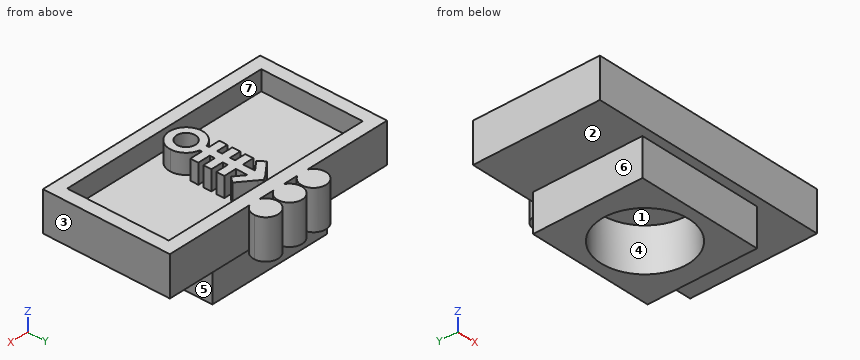
from build123d import *

# Parameters (mm, degrees)
F1_DEPTH = 3.175
F2_W     = 17.018
F2_H     = 8.128
F3_DEPTH = 1.5875
F4_W     = 10.05
F4_H     = 8.76
F5_DEPTH = 3
F6_R     = 3.5
F7_DEPTH = 3.5
F8_R     = 0.75
F8_W     = 0.64
F8_H     = 0.64
F8_W_2   = 1.0036083104
F8_W_3   = 0.8963916896
F8_H_2   = 0.4
F9_DEPTH = 1.5875


with BuildPart() as f1:
    # F0 (on Top) → F1 (new body)
    with BuildSketch(Plane.XY):
        with BuildLine():
            Line((-12.0608898944, 10.16), (-19.05, 10.16))
            Line((-19.05, 10.16), (-19.05, 0))
            Line((-19.05, 0), (0, 0))
            Line((0, 0), (0, 10.16))
            Line((0, 10.16), (-6.9891101056, 10.16))
            ThreePointArc((-6.9891101056, 10.16), (-7.425, 10.06), (-7.8608898944, 10.16))
            Line((-7.8608898944, 10.16), (-9.0891101056, 10.16))
            ThreePointArc((-9.0891101056, 10.16), (-9.525, 10.06), (-9.9608898944, 10.16))
            Line((-9.9608898944, 10.16), (-11.1891101056, 10.16))
            ThreePointArc((-11.1891101056, 10.16), (-11.625, 10.06), (-12.0608898944, 10.16))
        make_face()
        with BuildLine():
            ThreePointArc((-10.625, 11.06), (-12.1560885546, 11.9073163206), (-12.0608898944, 10.16))
            Line((-12.0608898944, 10.16), (-11.1891101056, 10.16))
            ThreePointArc((-11.1891101056, 10.16), (-10.7776836794, 10.5289114454), (-10.625, 11.06))
        make_face()
        with BuildLine():
            Line((-11.1891101056, 10.16), (-12.0608898944, 10.16))
            ThreePointArc((-12.0608898944, 10.16), (-11.625, 10.06), (-11.1891101056, 10.16))
        make_face()
        with BuildLine():
            ThreePointArc((-8.525, 11.06), (-10.0560885546, 11.9073163206), (-9.9608898944, 10.16))
            Line((-9.9608898944, 10.16), (-9.0891101056, 10.16))
            ThreePointArc((-9.0891101056, 10.16), (-8.6776836794, 10.5289114454), (-8.525, 11.06))
        make_face()
        with BuildLine():
            Line((-9.0891101056, 10.16), (-9.9608898944, 10.16))
            ThreePointArc((-9.9608898944, 10.16), (-9.525, 10.06), (-9.0891101056, 10.16))
        make_face()
        with BuildLine():
            ThreePointArc((-7.8608898944, 10.16), (-7.425, 10.06), (-6.9891101056, 10.16))
            Line((-6.9891101056, 10.16), (-7.8608898944, 10.16))
        make_face()
        with BuildLine():
            Line((-7.8608898944, 10.16), (-6.9891101056, 10.16))
            ThreePointArc((-6.9891101056, 10.16), (-6.5776836794, 10.5289114454), (-6.425, 11.06))
            ThreePointArc((-6.425, 11.06), (-7.9560885546, 11.9073163206), (-7.8608898944, 10.16))
        make_face()
    extrude(amount=F1_DEPTH)

    # F2 (on face) → F3 (cut)
    with BuildSketch(Plane.XY.offset(3.175)):
        with Locations((-9.525, 5.08)):
            Rectangle(F2_W, F2_H)
    extrude(amount=-F3_DEPTH, mode=Mode.SUBTRACT)

    # F4 (on face) → F5 (join)
    with BuildSketch(Plane(origin=(0, 0, 0), x_dir=(1, 0, 0), z_dir=(0, 0, -1))):
        with Locations((-9.525, -5.08)):
            Rectangle(F4_W, F4_H)
    extrude(amount=F5_DEPTH)

    # F6 (on face) → F7 (cut)
    with BuildSketch(Plane(origin=(0, 0, -3), x_dir=(1, 0, 0), z_dir=(0, 0, -1))):
        with Locations((-9.525, -5.08)):
            Circle(F6_R)
    extrude(amount=-F7_DEPTH, mode=Mode.SUBTRACT)

    # F8 (on face) → F9 (join, through all)
    with BuildSketch(Plane.XY.offset(1.5875)):
        with BuildLine():
            ThreePointArc((-9.8986083104, 4.0632728435), (-10.3368278084, 1.6873732761), (-8.175, 2.766))
            ThreePointArc((-8.175, 2.766), (-8.4804597229, 3.6212400888), (-9.2586083104, 4.0894558805))
            ThreePointArc((-9.2586083104, 4.0894558805), (-9.5801836824, 4.1148716622), (-9.8986083104, 4.0632728435))
        make_face()
        with Locations((-9.525, 2.766)):
            Circle(F8_R, mode=Mode.SUBTRACT)
        with BuildLine():
            ThreePointArc((-9.8986083104, 4.0632728435), (-9.5801836824, 4.1148716622), (-9.2586083104, 4.0894558805))
            Line((-9.2586083104, 4.0894558805), (-9.2586083104, 4.266))
            Line((-9.2586083104, 4.266), (-9.8986083104, 4.266))
            Line((-9.8986083104, 4.266), (-9.8986083104, 4.0632728435))
        make_face()
        with Locations((-9.5786083104, 4.586)):
            Rectangle(F8_W, F8_H)
        with Locations((-8.7568041552, 4.586)):
            Rectangle(F8_W_2, F8_H)
        with Locations((-10.3468041552, 4.586)):
            Rectangle(F8_W_3, F8_H)
        with Locations((-9.5786083104, 5.106)):
            Rectangle(F8_W, F8_H_2)
        with Locations((-9.5786083104, 5.626)):
            Rectangle(F8_W, F8_H)
        with Locations((-8.7568041552, 5.626)):
            Rectangle(F8_W_2, F8_H)
        with Locations((-10.3468041552, 5.626)):
            Rectangle(F8_W_3, F8_H)
        with Locations((-9.5786083104, 6.146)):
            Rectangle(F8_W, F8_H_2)
        with Locations((-9.5786083104, 6.666)):
            Rectangle(F8_W, F8_H)
        with Locations((-8.7568041552, 6.666)):
            Rectangle(F8_W_2, F8_H)
        with Locations((-10.3468041552, 6.666)):
            Rectangle(F8_W_3, F8_H)
        Polygon((-9.8986083104, 6.986), (-9.2586083104, 6.986), (-9.2586083104, 7.9498032218), (-9.2586083104, 8.763), (-9.8986083104, 8.763), (-9.8986083104, 7.9498032218), align=None)
        Polygon((-9.2586083104, 8.763), (-9.2586083104, 7.9498032218), (-8.4652456, 7.3151130535), (-8.0685642448, 7.8109647475), align=None)
        Polygon((-10.6919710208, 7.3151130535), (-9.8986083104, 7.9498032218), (-9.8986083104, 8.763), (-11.088652376, 7.8109647475), align=None)
        Polygon((-9.8986083104, 8.763), (-9.2586083104, 8.763), (-9.525, 8.9761133517), align=None)
    extrude(amount=F9_DEPTH)


solid = f1.part
Can you work these out from the model? Positions are in its coordinate system, mm. Face numbers are marked on the shaded views. A direction names the side the tool comes from. Round coordinates to 2 decimals unless told otherwise and drop trailing zeros. Order: outer loops, then holes, each group sorted by start corner. A loop starts at its lowest first (then second) coordinate and runs counter-clockwise, first axis right, second up. Notation, with made-up numbers: M 35.5,-21.75 L 53.5,-21.75 A33 cw 53.5,16.25 Z; hole C 18,88.25 d9. An arc over 180 degrees is marked long. Use a Markdown table: item, result.
1) On a 3-axis mill with a long thin cutter (end or side, diameter ignored), from which of +Z, -Z, +X, -X, +Y, -Y can I reach the whole of each face in a straight line? I mean the marked faces 4, 5, 6 and 7. Say none if no direction works.
Geometry says:
| item | result |
|---|---|
| face 4 | -Z |
| face 5 | -Z, +X, +Y, -Y |
| face 6 | -Z, -X, +Y, -Y |
| face 7 | +Z |
2) Imagine slicing it at C-C (z = -2.25). List the corners of the cut face in (x, y) for me (3 decimals), then the cut area to 3 significant figures.
Geometry says:
| item | result |
|---|---|
| outline | M -14.55,0.7 L -4.5,0.7 L -4.5,9.46 L -14.55,9.46 Z; hole C -9.525,5.08 d7 |
| area | 49.6 mm² |
3) Imagine slicing it at B-B (x = -4). List the corners of the cut face in (y, z) for me (1 decimal), then the cut area to 3 significant figures.
Geometry says:
| item | result |
|---|---|
| outline | M 0,0 L 10.2,0 L 10.2,3.2 L 9.1,3.2 L 9.1,1.6 L 1,1.6 L 1,3.2 L 0,3.2 Z |
| area | 19.4 mm² |
4) If we mould it in two halves opening along X, with no side actions, what happens to the marked faces 1, 2 and 3? For each: +X half, -X half, draft (parallel to the pull), parting line (faces both ways), or undercut.
Geometry says:
| item | result |
|---|---|
| face 1 | undercut |
| face 2 | draft |
| face 3 | +X half |
5) I'm going to push flat-ended pins straight in: P1, Ø1.5, axis at x = -10, z = -1, coming from the -Y side; P2, Ø0.9, axis at x = -9.5, z = -1, coming from the +Y side; P3, Ø0.9, axis at y = 7, z = -2, coming from the +X side. Where does each tip first touch, or does it pass through?
Geometry says:
| item | result |
|---|---|
| P1 | stops at y = 0.7 |
| P2 | stops at y = 9.46 |
| P3 | stops at x = -4.5 |
6) If I drill on line 1 along Y through (x, z) = (-5.5, 2.25); line 2 along X through (y, z) = (10.5, 1.25); line 3 along X through (y, z) = (5.08, -0.5) (3 decimals), over which ranges is the centre line in solid material (lowest first)?
Geometry says:
| item | result |
|---|---|
| line 1 | y = 0 to 1.02, 9.14 to 10.16 |
| line 2 | x = -12.45 to -10.8, -10.35 to -8.7, -8.25 to -6.6 |
| line 3 | x = -14.55 to -13.025, -6.025 to -4.5 |
7) Imagine slicing it at A-A (z = 1). List the corners of the cut face in (x, y) for me (3 decimals).
Geometry says:
| item | result |
|---|---|
| outline | M -19.05,0 L 0,0 L 0,10.16 L -6.989,10.16 A1 ccw long -7.861,10.16 L -9.089,10.16 A1 ccw long -9.961,10.16 L -11.189,10.16 A1 ccw long -12.061,10.16 L -19.05,10.16 Z |
